```python
from build123d import *

# Parameters (mm, degrees)
SKETCH1_W           = 100
SKETCH1_H           = 30
BOSS_EXTRUDE1_DEPTH = 2
SKETCH2_R           = 3
SKETCH2_R_2         = 1.5
CUT_EXTRUDE2_DEPTH  = 2


with BuildPart() as part:
    # Sketch1 → Boss-Extrude1 (new body)
    with BuildSketch(Plane.XY):
        with Locations((-27.462887989, 20.627530364)):
            Rectangle(SKETCH1_W, SKETCH1_H)
    boss_extrude1 = extrude(amount=BOSS_EXTRUDE1_DEPTH)

    # Sketch2 → Cut-Extrude2 (cut)
    with BuildSketch(Plane.XY.offset(2)):
        with Locations((-64.462887989, 20.196984479)):
            Circle(SKETCH2_R)
        with Locations((-72.962887989, 20.196984479)):
            Circle(SKETCH2_R_2)
        with Locations((-55.962887989, 20.196984479)):
            Circle(SKETCH2_R_2)
    cut_extrude2 = extrude(amount=-CUT_EXTRUDE2_DEPTH, mode=Mode.SUBTRACT)

    # Mirror2: Boss-Extrude1, Cut-Extrude2 across plane
    add(boss_extrude1.mirror(Plane(origin=(22.537112011, 35.627530364, 2), x_dir=(0, 0, 1), z_dir=(-1, 0, 0))))
    add(cut_extrude2.mirror(Plane(origin=(22.537112011, 35.627530364, 2), x_dir=(0, 0, 1), z_dir=(-1, 0, 0))), mode=Mode.SUBTRACT)


solid = part.part
```
Model file for the job. Use its own axes, mm. Round coordinates to 2 decimals unless told otherwise and drop trailing zeros. Use one line per item in the form item = value.
Item 1: Flat gauge pin, fed straight in: pin 1 Ø5 at (x, y) = (109.54, 20.2) entering from -Z. Where does the tip first touch, or does it go through?
Returned:
pin_1 = through
Item 2: Pull direction Y, two halves, no side cores. Call faces 1 (the face through (24, 21, 0)), 2 (the face through (-61.69, 19.05, 1.01)): released by +Y, released by -Y, zero draft, split by the parting line, or undercut.
Returned:
face_1 = zero draft
face_2 = undercut
Item 3: Drill centre lines: line 1 (X direction, y = 17.5, z = 1.15); line 2 (Y direction, x = -66.5, z = 1.55). Where is each one in solid material? Low to high.
Returned:
line_1 = -77.46 to -65.78, -63.15 to 108.22, 110.85 to 122.54
line_2 = 5.63 to 17.99, 22.4 to 35.63
